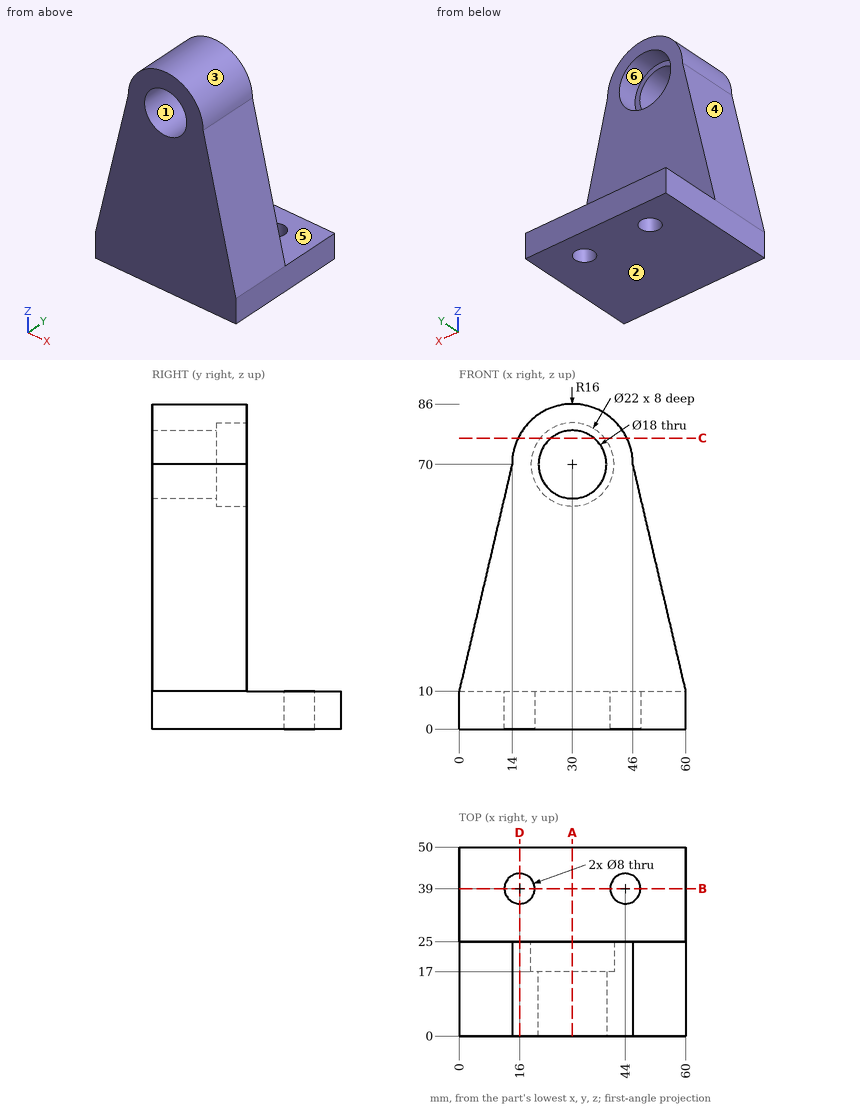
Geometry check sheet. Reference: drawing and pictorial views, mm from the part's lowest x, y, z. A direction names the side the tool comes from. Round coordinates to 2 decimals unless told otherwise and drop trailing zeros. Loops run counter-clockwise (first coordinate to the right, second up) from the corner with the lowest first, then second, coordinate; pieces in that order, holes last. Notation, with made-up numbers: (-20, 12) -> (36, 12) arc R25 cw to (36, 37) -> close; hole circle Ø9 at (24, -31). An arc over 180 degrees is marked (long way). Answer as a JSON object with one key per item and string values. Group by question number.
Item 1: Depth check by flat-ended pin: pin 1 Ø1.5 at (x, z) = (34.5, 41.5) entering from +Y; pin 2 Ø10 at (y, z) = (20.5, 50) entering from -X; pin 3 Ø10 at (y, z) = (12.5, 36) entering from -X; pin 4 Ø1 at (x, y) = (22, 21) entering from -Z. Enter the tip coordinate at first touch or a pass-through.
Item 2: Cross-section at B-B, the plane y = 39. Record the cut outline in (x, z), plus the area to 3 significant figures.
Item 3: Thickness scan on line 1 along Y through (x, z) = (44, 6); line 2 along Z through (x, y) = (30, 19); line 3 along Z through (x, y) = (47, 47). Record the ranges inside material, lowest first.
Item 4: Release check for a two-part mould opening along Z. For the marked faces 1, 2 and 3 record: pulls with the +Z half, pulls with the -Z half, needs draft (parallel to the pull), parting line crosses it, or undercut.
Item 5: Cross-section at A-A, the plane x = 30. Record the cut outline in (y, z).
Item 6: Cross-section at D-D, the plane x = 16. Record the cut outline in (y, z).
Item 7: Cross-section at C-C, the plane z = 77. Record the cut outline in (x, y).
Item 8: Set-up check for the marked faces 4, 5 and 6: record each of +Z, -Z, +X, -X, +Y, -Y from which the full face is reachable in a straight line by a thin tool's end or side.
Determined:
{
 "1": {"pin 1": "stops at y = 25", "pin 2": "stops at x = 8.17", "pin 3": "stops at x = 4.9", "pin 4": "stops at z = 0"},
 "2": {"outline": "(0, 0) -> (12, 0) -> (12, 10) -> (0, 10) -> close; (20, 0) -> (40, 0) -> (40, 10) -> (20, 10) -> close; (48, 0) -> (60, 0) -> (60, 10) -> (48, 10) -> close", "area": "440 mm²"},
 "3": {"line 1": "y = 0 to 35, 43 to 50", "line 2": "z = 0 to 59, 81 to 86", "line 3": "z = 0 to 10"},
 "4": {"face 1": "undercut", "face 2": "pulls with the -Z half", "face 3": "pulls with the +Z half"},
 "5": {"outline": "(0, 0) -> (50, 0) -> (50, 10) -> (25, 10) -> (25, 59) -> (17, 59) -> (17, 61) -> (0, 61) -> close; (0, 79) -> (17, 79) -> (17, 81) -> (25, 81) -> (25, 86) -> (0, 86) -> close"},
 "6": {"outline": "(0, 0) -> (35, 0) -> (35, 10) -> (25, 10) -> (25, 77.75) -> (0, 77.75) -> close; (43, 0) -> (50, 0) -> (50, 10) -> (43, 10) -> close"},
 "7": {"outline": "(15.61, 0) -> (24.34, 0) -> (24.34, 17) -> (21.51, 17) -> (21.51, 25) -> (15.61, 25) -> close; (35.66, 0) -> (44.39, 0) -> (44.39, 25) -> (38.49, 25) -> (38.49, 17) -> (35.66, 17) -> close"},
 "8": {"face 4": "+Z, -X, +Y, -Y", "face 5": "+Z, +X, -X, +Y", "face 6": "+Y"}
}
